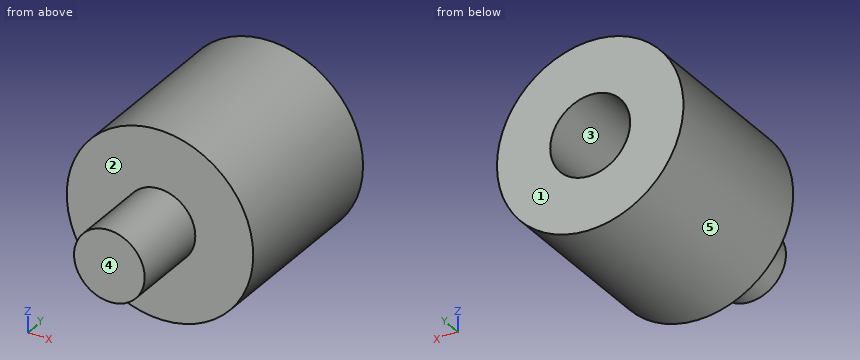
```python
from build123d import *

# Parameters (mm, degrees)
SKETCH1_R           = 1.325
BOSS_EXTRUDE1_DEPTH = 3
SKETCH2_R           = 3.5
BOSS_EXTRUDE2_DEPTH = 1.5
SKETCH3_R           = 3.5
SKETCH3_R_2         = 1.5
BOSS_EXTRUDE3_DEPTH = 5


with BuildPart() as part:
    # Sketch1 → Boss-Extrude1 (new body)
    with BuildSketch(Plane(origin=(0, 0, 0), x_dir=(1, 0, 0), z_dir=(0, 1, 0))):
        Circle(SKETCH1_R)
    extrude(amount=BOSS_EXTRUDE1_DEPTH)

    # Sketch2 → Boss-Extrude2 (add)
    with BuildSketch(Plane(origin=(0, 3, 0), x_dir=(1, 0, 0), z_dir=(0, 1, 0))):
        Circle(SKETCH2_R)
    extrude(amount=BOSS_EXTRUDE2_DEPTH)

    # Sketch3 → Boss-Extrude3 (add)
    with BuildSketch(Plane(origin=(0, 4.5, 0), x_dir=(1, 0, 0), z_dir=(0, 1, 0))):
        Circle(SKETCH3_R)
        Circle(SKETCH3_R_2, mode=Mode.SUBTRACT)
    extrude(amount=BOSS_EXTRUDE3_DEPTH)


solid = part.part
```
CAD build for the part. Positions are in the model's coordinates, mm. Face numbers are marked on the shaded views. A direction names the side the tool comes from. Round coordinates to 2 decimals unless told otherwise and drop trailing zeros. Write each loop counter-clockwise with the first axis right and the second up, starting at its lowest first coordinate (ties: lowest second). Pieces come first, ordered by that corner, then holes. Notation, with made-up numbers: (50.5, 69.25) - (74.5, 69.25) arc R19 ccw to (74.5, 83.25) - close; hole circle Ø7 at (47.25, 23). An arc over 180 degrees is marked (long way). Return JSON: item names as keys, results as strings. Group by question number.
Item 1: Band-saw the part on A-A on z = 0. List the corners of the cut face in (x, y) (3 decimals).
Item 2: Probe probe 1 along X at (y, z) = (5.8, 0); probe 2 along Y at (x, z) = (2.25, 0). List the from-to ranges inside material, lowest first.
Item 3: Band-saw the part on B-B on x = 0. List the corners of the cut face in (y, z) (3 decimals), plus the area to 4 significant figures.
Item 4: Band-saw the part on D-D on y = 2. List the corners of the cut face in (x, z) (3 decimals).
Item 5: Mould opens along X. For the marked faces 3, 4 and 5 say: +X half, -X half, draft (parallel to the pull), parting line (faces both ways), or undercut.
Item 6: Band-saw the part on C-C on y = 6.75. List the corners of the cut face in (x, z), plus the area to 3 significant figures.
Item 7: Flat gauge pins, fed straight in: pin 1 Ø0.9 at (x, z) = (-0.5, 0) entering from +Y; pin 2 Ø2 at (x, y) = (0.5, 1) entering from +Z (3 decimals); pin 3 Ø2 at (y, z) = (1.5, -0.5) entering from +X (3 decimals). Where does each tip first touch, or does it go through?
Item 8: 3-axis set-ups, long thin cutter, end or side, ignore diameter. For the marked faces 1 and 2: which of +Z, -Z, +X, -X, +Y, -Y reach the whole face in a straight line?
Resolved:
{
 "1": {"outline": "(-3.5, 3) - (-1.325, 3) - (-1.325, 0) - (1.325, 0) - (1.325, 3) - (3.5, 3) - (3.5, 9.5) - (1.5, 9.5) - (1.5, 4.5) - (-1.5, 4.5) - (-1.5, 9.5) - (-3.5, 9.5) - close"},
 "2": {"probe 1": "x = -3.5 to -1.5, 1.5 to 3.5", "probe 2": "y = 3 to 9.5"},
 "3": {"outline": "(0, -1.325) - (3, -1.325) - (3, -3.5) - (9.5, -3.5) - (9.5, -1.5) - (4.5, -1.5) - (4.5, 1.5) - (9.5, 1.5) - (9.5, 3.5) - (3, 3.5) - (3, 1.325) - (0, 1.325) - close", "area": "38.45 mm²"},
 "4": {"outline": "circle Ø2.65 at (0, 0)"},
 "5": {"face 3": "undercut", "face 4": "draft", "face 5": "parting line"},
 "6": {"outline": "circle Ø7 at (0, 0); hole circle Ø3 at (0, 0)", "area": "31.4 mm²"},
 "7": {"pin 1": "stops at y = 4.5", "pin 2": "stops at z = 1.325", "pin 3": "stops at x = 1.325"},
 "8": {"face 1": "+Z, -Z, +X, -X, +Y", "face 2": "-Y"}
}
